Source: CAD feature listing. Evaluate the final solid. Frame: model axes, mm. Face numbers are marked on the shaded views. A direction names the side the tool comes from. Coordinates: 2 decimals unless noted, no trailing zeros. Order: outer loops, then holes, each group sorted by start corner. A loop starts at its lowest first (then second) coordinate and runs counter-clockwise, first axis right, second up. Notation, with made-up numbers: (28.5, 55.5) -> (37.5, 55.5) arc R20 cw to (37.5, 90.5) -> close; hole circle Ø9 at (-24, -9.5). An arc over 180 degrees is marked (long way). Write item = value, one per line. Start each with the question number.
Item 1: Set-up query: the marked faces 1, 2, 3 and 4. Return all of +Z, -Z, +X, -X, +Y, -Y with unobstructed straight access to the full face (end or side cutting, diameter ignored); none if empty.
Item 2: Section query C-C (z = 58.5). Output: boundary loops of the cut face in (x, y), then the cut area to 3 significant figures.
Item 3: Contact query for flat-ended pins moving along their axis: pin 1 (4 mm diameter, centred on x = 1.5, y = -30, fed in from -Z); pin 2 (6.5 mm diameter, centred on x = -0.5, y = -25, fed in from +Z). Output: stop coordinate, or through.
Item 4: Section query A-A (x = 0). Output: boundary loops of the cut face in (y, z).
Item 5: Ray query, line 1 along X through (y, z) = (-33.25, 65.5); line 2 along Y through (x, z) = (-5, 54). Return the intervals inside material, ascending. Write a range as [from, to].
Item 6: Mould query, pull axis Y, two halves, no side actions, for the marked faces 5, 6, 7 and 8. Classes: released by +Y, released by -Y, zero draft, split by the parting line, or undercut.
Item 7: Section query B-B (y = -30.75). Output: boundary loops of the cut face in (x, z), then the cut area to 3 significant figures.
Item 8: Section query D-D (x = 8.5). Output: boundary loops of the cut face in (y, z).
```python
from build123d import *

# Parameters (mm, degrees)
F0_W     = 24.5
F0_H     = 24.5
F1_DEPTH = 37
F2_DEPTH = 20
F3_DEPTH = 3
F5_DEPTH = 2.7
F6_R     = 2
F7_ANGLE = -180


with BuildPart() as f1:
    # F0 (on Top) → F1 (new body)
    with BuildSketch(Plane.XY):
        Rectangle(F0_W, F0_H)
        Polygon((10.25, -3), (10.25, -10.25), (3, -10.25), (-3, -10.25), (-10.25, -10.25), (-10.25, -3), (-10.25, 3), (-10.25, 10.25), (-3, 10.25), (3, 10.25), (10.25, 10.25), (10.25, 3), align=None, mode=Mode.SUBTRACT)
    extrude(amount=F1_DEPTH)

    # F0 (on Top) → F2 (join)
    with BuildSketch(Plane.XY):
        Rectangle(F0_W, F0_H)
        Polygon((10.25, -3), (10.25, -10.25), (3, -10.25), (-3, -10.25), (-10.25, -10.25), (-10.25, -3), (-10.25, 3), (-10.25, 10.25), (-3, 10.25), (3, 10.25), (10.25, 10.25), (10.25, 3), align=None, mode=Mode.SUBTRACT)
        with BuildLine():
            Line((-3, -10.25), (3, -10.25))
            ThreePointArc((3, -10.25), (0, -7.25), (-3, -10.25))
        make_face()
        with BuildLine():
            Line((-10.25, 3), (-10.25, -3))
            ThreePointArc((-10.25, -3), (-7.25, 0), (-10.25, 3))
        make_face()
        with BuildLine():
            ThreePointArc((10.25, 3), (7.25, 0), (10.25, -3))
            Line((10.25, -3), (10.25, 3))
        make_face()
    extrude(amount=-F2_DEPTH)

    # F0 (on Top) → F3 (join)
    with BuildSketch(Plane.XY):
        with BuildLine():
            Line((3, -10.25), (10.25, -10.25))
            Line((10.25, -10.25), (10.25, -3))
            ThreePointArc((10.25, -3), (7.25, 0), (10.25, 3))
            Line((10.25, 3), (10.25, 10.25))
            Line((10.25, 10.25), (3, 10.25))
            ThreePointArc((3, 10.25), (0, 7.25), (-3, 10.25))
            Line((-3, 10.25), (-10.25, 10.25))
            Line((-10.25, 10.25), (-10.25, 3))
            ThreePointArc((-10.25, 3), (-7.25, 0), (-10.25, -3))
            Line((-10.25, -3), (-10.25, -10.25))
            Line((-10.25, -10.25), (-3, -10.25))
            ThreePointArc((-3, -10.25), (0, -7.25), (3, -10.25))
        make_face()
        with BuildLine():
            Line((-10.25, 3), (-10.25, -3))
            ThreePointArc((-10.25, -3), (-7.25, 0), (-10.25, 3))
        make_face()
        with BuildLine():
            Line((-3, -10.25), (3, -10.25))
            ThreePointArc((3, -10.25), (0, -7.25), (-3, -10.25))
        make_face()
        with BuildLine():
            ThreePointArc((10.25, 3), (7.25, 0), (10.25, -3))
            Line((10.25, -3), (10.25, 3))
        make_face()
    extrude(amount=F3_DEPTH)

    # F4 (on face) → F5 (cut)
    with BuildSketch(Plane(origin=(0, 0, 0), x_dir=(1, 0, 0), z_dir=(0, 0, -1))):
        with BuildLine():
            Line((3, -10.25), (3, 0))
            ThreePointArc((3, 0), (0, -3), (-3, 0))
            Line((-3, 0), (-3, -10.25))
            ThreePointArc((-3, -10.25), (0, -7.25), (3, -10.25))
        make_face()
        with BuildLine():
            ThreePointArc((-3, 0), (0, -3), (3, 0))
            ThreePointArc((3, 0), (0, 3), (-3, 0))
        make_face()
    extrude(amount=-F5_DEPTH, mode=Mode.SUBTRACT)

    # F6
    f6_edges = [f1.edges().sort_by_distance(p)[0] for p in [
        (-12.25, -12.25, 8.5),
        (12.25, -12.25, 8.5),
        (12.25, 12.25, 8.5),
        (-12.25, 12.25, 8.5),
    ]]
    fillet(f6_edges, radius=F6_R)


with BuildPart() as f1_1:
    # F7: moved
    add(f1.part.rotate(Axis((0, -12.25, 37), (-1, 0, 0)), F7_ANGLE))


solid = f1_1.part
```
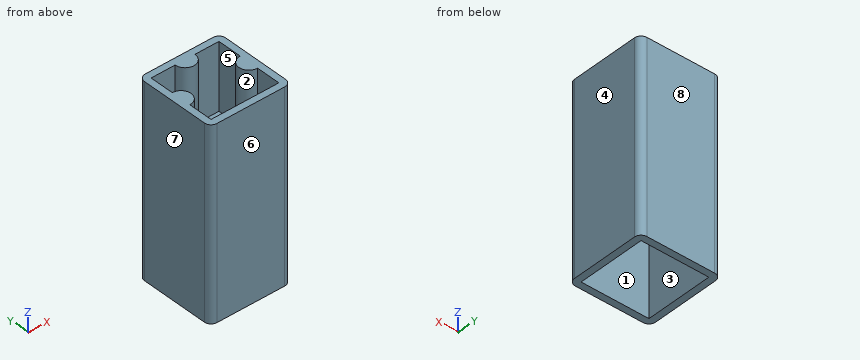
Computed:
q1.face_1 = none
q1.face_2 = +Z
q1.face_3 = -Z
q1.face_4 = +Z, -Z, +X, +Y, -Y
q2.outline = (-12.25, -34.75) arc R2 ccw to (-10.25, -36.75) -> (10.25, -36.75) arc R2 ccw to (12.25, -34.75) -> (12.25, -14.25) arc R2 ccw to (10.25, -12.25) -> (-10.25, -12.25) arc R2 ccw to (-12.25, -14.25) -> close; hole (-10.25, -34.75) -> (10.25, -34.75) -> (10.25, -14.25) -> (-10.25, -14.25) -> close
q2.area = 177 mm^2
q3.pin_1 = 71
q3.pin_2 = 74
q4.outline = (-36.75, 37) -> (-34.75, 37) -> (-34.75, 94) -> (-36.75, 94) -> close; (-31.75, 71) -> (-14.25, 71) -> (-14.25, 37) -> (-12.25, 37) -> (-12.25, 94) -> (-17.25, 94) -> (-17.25, 74) -> (-21.5, 74) -> (-21.5, 71.3) -> (-31.75, 71.3) -> close
q5.line_1 = [-12.25, -10.25], [10.25, 12.25]
q5.line_2 = [-36.75, -34.75], [-14.25, -12.25]
q6.face_5 = undercut
q6.face_6 = released by -Y
q6.face_7 = zero draft
q6.face_8 = released by +Y
q7.outline = (-12.25, 37) -> (-10.25, 37) -> (-10.25, 71) -> (10.25, 71) -> (10.25, 37) -> (12.25, 37) -> (12.25, 94) -> (10.25, 94) -> (10.25, 74) -> (3, 74) -> (3, 71.3) -> (-3, 71.3) -> (-3, 74) -> (-10.25, 74) -> (-10.25, 94) -> (-12.25, 94) -> close
q7.area = 273 mm^2
q8.outline = (-36.75, 37) -> (-34.75, 37) -> (-34.75, 71) -> (-14.25, 71) -> (-14.25, 37) -> (-12.25, 37) -> (-12.25, 94) -> (-14.25, 94) -> (-14.25, 74) -> (-22.06, 74) -> (-22.06, 94) -> (-26.94, 94) -> (-26.94, 74) -> (-34.75, 74) -> (-34.75, 94) -> (-36.75, 94) -> close
